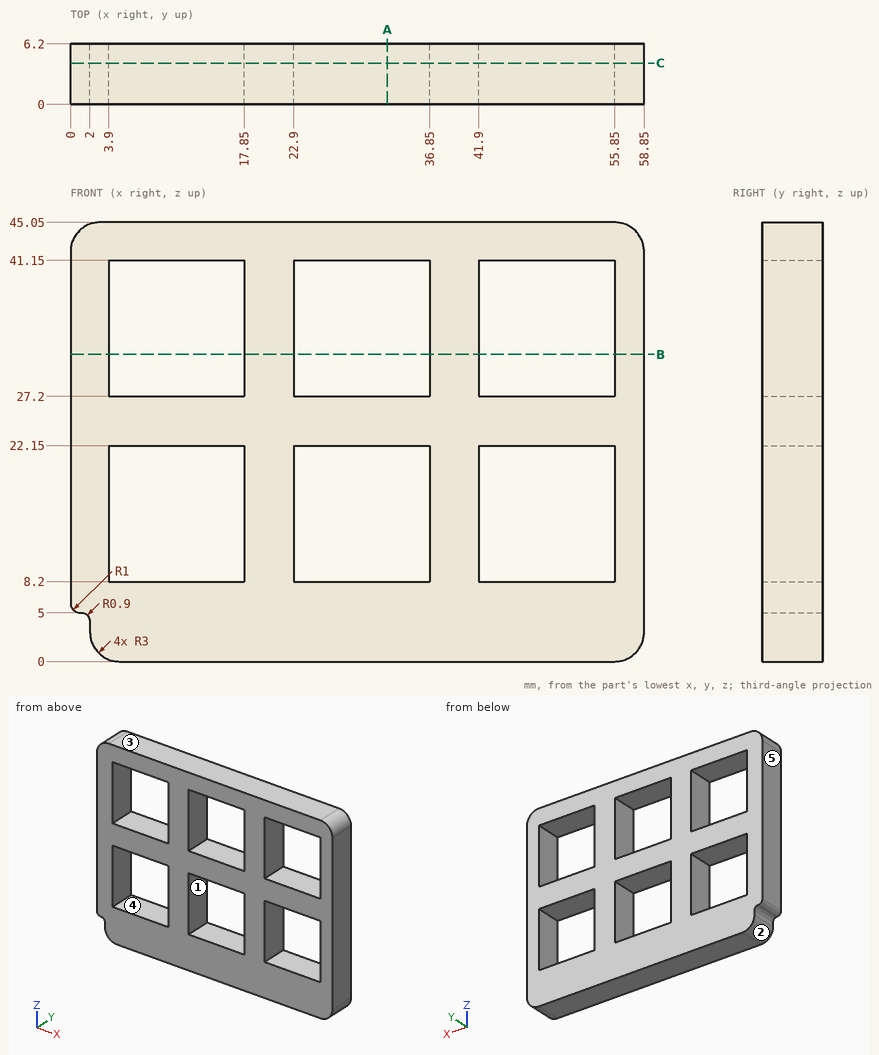
Source: three-view drawing plus pictorial views. Frame: mm from the lowest corner of the part. A direction names the side the tool comes from. Coordinates: 2 decimals unless noted, no trailing zeros. Order: outer loops, then holes, each group sorted by start corner. A loop starts at its lowest first (then second) coordinate and runs counter-clockwise, first axis right, second up. Notation, with made-up numbers: M 86,-9 L 113,-9 A29 ccw 113,28 Z; hole C -34,82.25 d5. An arc over 180 degrees is marked long. One line per question, with ' | ' between items. Start each with the question number.
Item 1: Ray query, probe 1 along X at (y, z) = (1, 35); probe 2 along Z at (x, y) = (36.5, 3.75); probe 3 along X at (y, z) = (5.25, 3). Return the intervals inside material, ascending. Write a range as [from, to].
Item 2: Set-up query: the marked faces 4 and 5. Return all of +Z, -Z, +X, -X, +Y, -Y with unobstructed straight access to the full face (end or side cutting, diameter ignored); none if empty.
Item 3: Cut plane B-B, the plane z = 31.5. Return the cut outline in (x, y), then the cut area to 3 significant figures.
Item 4: Cut plane A-A, the plane x = 32.5. Return the cut outline in (y, z).
Item 5: Draft query along X for the marked faces 1, 2 and 3. Return one class per face: released by +X, released by -X, zero draft, split by the parting line, or undercut.
Item 6: Cut plane C-C, the plane y = 4.25. Count the separate pieces of the cut face and the enclosed holes in it, then the cut area to 3 significant figures.
A:
1) probe 1: x = [0, 3.9], [17.85, 22.9], [36.85, 41.9], [55.85, 58.85] | probe 2: z = [0, 8.2], [22.15, 27.2], [41.15, 45.05] | probe 3: x = [2, 58.85]
2) face 4: +Y, -Y | face 5: +Z, -Z, -X, +Y, -Y
3) outline: M 0,0 L 3.9,0 L 3.9,6.2 L 0,6.2 Z; M 17.85,0 L 22.9,0 L 22.9,6.2 L 17.85,6.2 Z; M 36.85,0 L 41.9,0 L 41.9,6.2 L 36.85,6.2 Z; M 55.85,0 L 58.85,0 L 58.85,6.2 L 55.85,6.2 Z | area: 105 mm2
4) outline: M 0,0 L 6.2,0 L 6.2,8.2 L 0,8.2 Z; M 0,22.15 L 6.2,22.15 L 6.2,27.2 L 0,27.2 Z; M 0,41.15 L 6.2,41.15 L 6.2,45.05 L 0,45.05 Z
5) face 1: undercut | face 2: released by -X | face 3: zero draft
6) separate pieces: 1 | enclosed holes: 6 | area: 1,470 mm2
